```python
from build123d import *

# Parameters (mm, degrees)
SCHIZZO1_R                                           = 110.5
SCHIZZO1_R_2                                         = 103
ESTRUSIONE_ESTRUSIONE1_DEPTH                         = 150
FORO_LAMATO_PER_BULLONE_M12_A_TESTA_ESAG_D           = 5.4
FORO_LAMATO_PER_BULLONE_M12_A_TESTA_ESAG_DEPTH       = 8.1
FORO_LAMATO_PER_BULLONE_M12_A_TESTA_ESAG_CBORE_D     = 10
FORO_LAMATO_PER_BULLONE_M12_A_TESTA_ESAG_CBORE_DEPTH = 3
FORO_LAMATO_PER_BULLONE_M12_A_TESTA_ESAG_TIP         = 1.622323671
FORO_LAMATO_PER_BULLONE_M12_A_TESTA_2_D              = 5.4
FORO_LAMATO_PER_BULLONE_M12_A_TESTA_2_DEPTH          = 8.1
FORO_LAMATO_PER_BULLONE_M12_A_TESTA_2_CBORE_D        = 10
FORO_LAMATO_PER_BULLONE_M12_A_TESTA_2_CBORE_DEPTH    = 3
FORO_LAMATO_PER_BULLONE_M12_A_TESTA_2_TIP            = 1.622323671
FORO_LAMATO_PER_BULLONE_M12_A_TESTA_3_D              = 5.4
FORO_LAMATO_PER_BULLONE_M12_A_TESTA_3_DEPTH          = 8.1
FORO_LAMATO_PER_BULLONE_M12_A_TESTA_3_CBORE_D        = 10
FORO_LAMATO_PER_BULLONE_M12_A_TESTA_3_CBORE_DEPTH    = 3
FORO_LAMATO_PER_BULLONE_M12_A_TESTA_3_TIP            = 1.622323671
FORO_LAMATO_PER_BULLONE_M12_A_TESTA_4_D              = 5.4
FORO_LAMATO_PER_BULLONE_M12_A_TESTA_4_DEPTH          = 8.1
FORO_LAMATO_PER_BULLONE_M12_A_TESTA_4_CBORE_D        = 10
FORO_LAMATO_PER_BULLONE_M12_A_TESTA_4_CBORE_DEPTH    = 3
FORO_LAMATO_PER_BULLONE_M12_A_TESTA_4_TIP            = 1.622323671
SCHIZZO4_R                                           = 103
SCHIZZO4_R_2                                         = 73
ESTRUSIONE_ESTRUSIONE2_DEPTH                         = 5
FORO_PER_VITE_M6_1_D                                 = 6.6


with BuildPart() as part:
    # Schizzo1 → Estrusione-Estrusione1 (new body)
    with BuildSketch(Plane(origin=(0, 0, 0), x_dir=(1, 0, 0), z_dir=(0, 1, 0))):
        with Locations(Location((0, 0, 0), (0, 0, 270))):
            Circle(SCHIZZO1_R)
        with Locations(Location((0, 0, 0), (0, 0, 270))):
            Circle(SCHIZZO1_R_2, mode=Mode.SUBTRACT)
    extrude(amount=ESTRUSIONE_ESTRUSIONE1_DEPTH)

    # Foro lamato per Bullone M12 a testa esagonale (Classe superiore)-1
    with Locations(Plane(origin=(0, 140, 110.5), x_dir=(1, 0, 0), z_dir=(0, 0, 1))):
        with Locations((0, 0)):
            CounterBoreHole(FORO_LAMATO_PER_BULLONE_M12_A_TESTA_ESAG_D / 2, FORO_LAMATO_PER_BULLONE_M12_A_TESTA_ESAG_CBORE_D / 2, FORO_LAMATO_PER_BULLONE_M12_A_TESTA_ESAG_CBORE_DEPTH, depth=FORO_LAMATO_PER_BULLONE_M12_A_TESTA_ESAG_DEPTH)
            with Locations((0, 0, -(FORO_LAMATO_PER_BULLONE_M12_A_TESTA_ESAG_DEPTH + FORO_LAMATO_PER_BULLONE_M12_A_TESTA_ESAG_TIP / 2))):  # 118° drill point
                Cone(0, FORO_LAMATO_PER_BULLONE_M12_A_TESTA_ESAG_D / 2, FORO_LAMATO_PER_BULLONE_M12_A_TESTA_ESAG_TIP, mode=Mode.SUBTRACT)

    # Foro lamato per Bullone M12 a testa  2
    with Locations(Plane(origin=(110.5, 140, 0), x_dir=(0, 0, 1), z_dir=(1, 0, 0))):
        with Locations((0, 0)):
            CounterBoreHole(FORO_LAMATO_PER_BULLONE_M12_A_TESTA_2_D / 2, FORO_LAMATO_PER_BULLONE_M12_A_TESTA_2_CBORE_D / 2, FORO_LAMATO_PER_BULLONE_M12_A_TESTA_2_CBORE_DEPTH, depth=FORO_LAMATO_PER_BULLONE_M12_A_TESTA_2_DEPTH)
            with Locations((0, 0, -(FORO_LAMATO_PER_BULLONE_M12_A_TESTA_2_DEPTH + FORO_LAMATO_PER_BULLONE_M12_A_TESTA_2_TIP / 2))):  # 118° drill point
                Cone(0, FORO_LAMATO_PER_BULLONE_M12_A_TESTA_2_D / 2, FORO_LAMATO_PER_BULLONE_M12_A_TESTA_2_TIP, mode=Mode.SUBTRACT)

    # Foro lamato per Bullone M12 a testa  3
    with Locations(Plane(origin=(0, 140, -110.5), x_dir=(-1, 0, 0), z_dir=(0, 0, -1))):
        with Locations((0, 0)):
            CounterBoreHole(FORO_LAMATO_PER_BULLONE_M12_A_TESTA_3_D / 2, FORO_LAMATO_PER_BULLONE_M12_A_TESTA_3_CBORE_D / 2, FORO_LAMATO_PER_BULLONE_M12_A_TESTA_3_CBORE_DEPTH, depth=FORO_LAMATO_PER_BULLONE_M12_A_TESTA_3_DEPTH)
            with Locations((0, 0, -(FORO_LAMATO_PER_BULLONE_M12_A_TESTA_3_DEPTH + FORO_LAMATO_PER_BULLONE_M12_A_TESTA_3_TIP / 2))):  # 118° drill point
                Cone(0, FORO_LAMATO_PER_BULLONE_M12_A_TESTA_3_D / 2, FORO_LAMATO_PER_BULLONE_M12_A_TESTA_3_TIP, mode=Mode.SUBTRACT)

    # Foro lamato per Bullone M12 a testa  4
    with Locations(Plane(origin=(-110.5, 140, 0), x_dir=(0, 0, -1), z_dir=(-1, 0, 0))):
        with Locations((0, 0)):
            CounterBoreHole(FORO_LAMATO_PER_BULLONE_M12_A_TESTA_4_D / 2, FORO_LAMATO_PER_BULLONE_M12_A_TESTA_4_CBORE_D / 2, FORO_LAMATO_PER_BULLONE_M12_A_TESTA_4_CBORE_DEPTH, depth=FORO_LAMATO_PER_BULLONE_M12_A_TESTA_4_DEPTH)
            with Locations((0, 0, -(FORO_LAMATO_PER_BULLONE_M12_A_TESTA_4_DEPTH + FORO_LAMATO_PER_BULLONE_M12_A_TESTA_4_TIP / 2))):  # 118° drill point
                Cone(0, FORO_LAMATO_PER_BULLONE_M12_A_TESTA_4_D / 2, FORO_LAMATO_PER_BULLONE_M12_A_TESTA_4_TIP, mode=Mode.SUBTRACT)

    # Schizzo4 → Estrusione-Estrusione2 (add)
    with BuildSketch(Plane.XZ):
        with Locations(Location((0, 0, 0), (0, 0, 270))):
            Circle(SCHIZZO4_R)
        with Locations(Location((0, 0, 0), (0, 0, 270))):
            Circle(SCHIZZO4_R_2, mode=Mode.SUBTRACT)
    extrude(amount=-ESTRUSIONE_ESTRUSIONE2_DEPTH)

    # Foro per Vite M6-1 (through all)
    with Locations(Plane(origin=(0, 5, 0), x_dir=(1, 0, 0), z_dir=(0, 1, 0))):
        with Locations((0, -88), (-88, 0), (88, 0), (0, 88)):
            Hole(FORO_PER_VITE_M6_1_D / 2)


solid = part.part
```
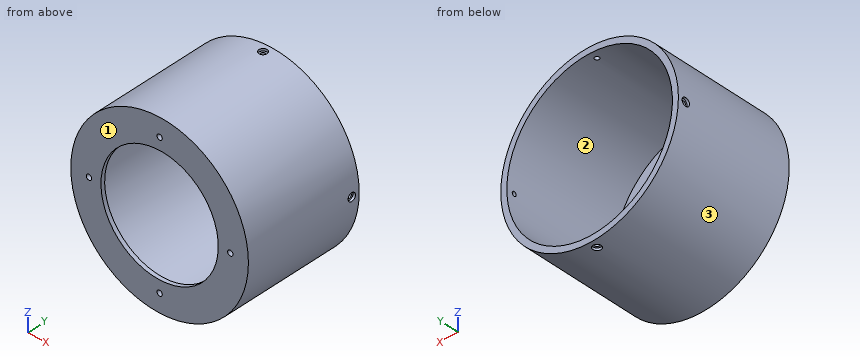
Geometry check sheet. Reference: the model listing, model coordinates, mm. Face numbers are marked on the shaded views. Give positions to 0.01 mm unless a question says otherwise; leave off trailing zeros. Order: outer loops, then holes, each group sorted by start corner. A loop starts at its lowest first (then second) coordinate and runs counter-clockwise, first axis right, second up.
1. Thickness scan on L1, parallel to X at y = 15.5, z = -1; L2, parallel to Y at x = -97, z = 30.5; L3, parallel to X at y = 33, z = -52.5. Record the ranges inside material, lowest first.
2. Section check A-A, the plane z = -64.5. Enter the section's corners in (x, y).
3. Gauge pin test, flat ends, axial feed: pin 1 Ø8 at (y, z) = (139.5, 0.5) entering from +X; pin 2 Ø6 at (x, y) = (-9, 42.5) entering from -Z; pin 3 Ø8 at (x, y) = (41, 76.5) entering from +Z. Record the tip position at first contact, or that the pin passes through.
4. Release check for a two-part mould opening along Z. For the marked faces 1, 2 and 3 record: pulls with the +Z half, pulls with the -Z half, needs draft (parallel to the pull), parting line crosses it, or undercut.
5. Section check C-C, the plane y = 25.5. Enter the section's corners in (x, z).
6. Section check B-B, the plane x = 29. Enter the section's corners in (y, z), and give its area (3 significant figures).
Values follow:
1. L1: x = -110.5 to -103, 103 to 110.5
1. L2: y = 0 to 5
1. L3: x = -97.23 to -88.62, 88.62 to 97.23
2. outline: (-89.72, 0) - (-34.19, 0) - (-34.19, 5) - (-80.3, 5) - (-80.3, 150) - (-89.72, 150) - close; (34.19, 0) - (89.72, 0) - (89.72, 150) - (80.3, 150) - (80.3, 5) - (34.19, 5) - close
3. pin 1: stops at x = 107.5
3. pin 2: stops at z = -110.34
3. pin 3: stops at z = 104.12
4. face 1: needs draft
4. face 2: undercut
4. face 3: parting line crosses it
5. outline: circle Ø221 at (0, 0); hole circle Ø206 at (0, 0)
6. outline: (0, -106.63) - (150, -106.63) - (150, -98.83) - (5, -98.83) - (5, -66.99) - (0, -66.99) - close; (0, 66.99) - (5, 66.99) - (5, 98.83) - (150, 98.83) - (150, 106.63) - (0, 106.63) - close
6. area: 2,660 mm2
